Source: three-view drawing plus pictorial views. Frame: mm from the lowest corner of the part. A direction names the side the tool comes from. Give positions to 0.01 mm unless a question says otherwise; leave off trailing zeros. Order: outer loops, then holes, each group sorted by start corner. A loop starts at its lowest first (then second) coordinate and runs counter-clockwise, first axis right, second up.
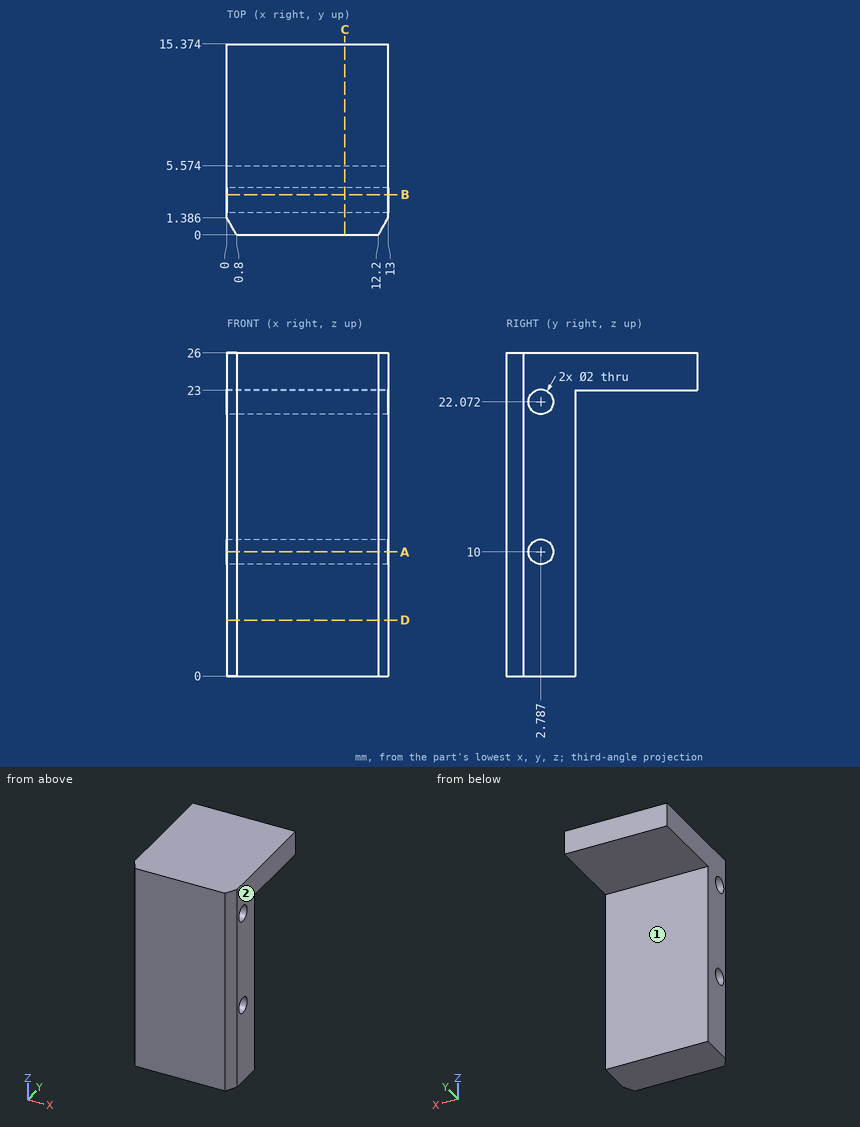
1) Section query C-C on x = 9.5. Output: boundary loops of the cut face in (y, z).
Checks:
outline: (0, 0) - (5.57, 0) - (5.57, 23) - (15.37, 23) - (15.37, 26) - (0, 26) - close; hole circle Ø2 at (2.79, 10); hole circle Ø2 at (2.79, 22.07)
2) Section query B-B on y = 3.25. Output: boundary loops of the cut face in (x, z) (1 decimal).
Checks:
outline: (0, 0) - (13, 0) - (13, 9.1) - (0, 9.1) - close; (0, 10.9) - (13, 10.9) - (13, 21.2) - (0, 21.2) - close; (0, 23) - (13, 23) - (13, 26) - (0, 26) - close
3) Section query D-D on z = 4.5. Output: boundary loops of the cut face in (x, y) (1 decimal).
Checks:
outline: (0, 1.4) - (0.8, 0) - (12.2, 0) - (13, 1.4) - (13, 5.6) - (0, 5.6) - close
4) First-contact query: pin 1 Ø6 at (x, z) = (8.5, 13.5) entering from +Y; pin 2 Ø4 at (x, y) = (6.5, 8.5) entering from -Z. Flat tips, straight axial feed; report the tip coordinate or a pass-through.
Checks:
pin 1: stops at y = 5.57
pin 2: stops at z = 23
5) Reachability of the marked faces 1 and 2 from +Z, -Z, +X, -X, +Y, -Y: full face, straight path, thin tool, end or side. Return the list, or none.
Checks:
face 1: -Z, +X, -X, +Y
face 2: +Z, -Z, +X, +Y, -Y
6) Ray query, L1, parallel to Y at x = 6.5, z = 10; L2, parallel to Z at x = 12, y = 2 (1 decimal); L3, parallel to Z at x = 2.5, y = 14.75. Return the intervals inside material, ascending.
Checks:
L1: y = 0 to 1.79, 3.79 to 5.57
L2: z = 0 to 9.4, 10.6 to 21.5, 22.7 to 26
L3: z = 23 to 26
7) Section query A-A on z = 10. Output: boundary loops of the cut face in (x, y) (1 decimal).
Checks:
outline: (0, 1.4) - (0.8, 0) - (12.2, 0) - (13, 1.4) - (13, 1.8) - (0, 1.8) - close; (0, 3.8) - (13, 3.8) - (13, 5.6) - (0, 5.6) - close
